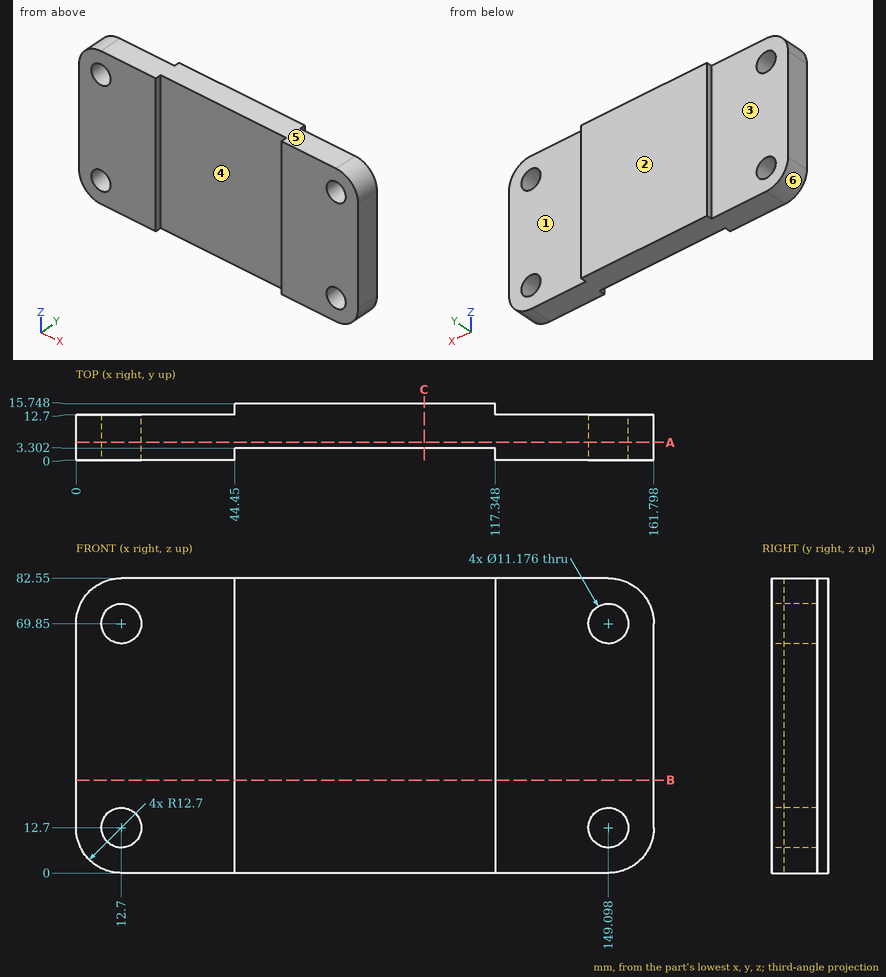
Print and shaded views of the part. All mm, measured from the part's lowest x, y and z. A direction names the side the tool comes from. Give positions to 0.01 mm unless a question says otherwise; leave off trailing zeros. Write each loop counter-clockwise with the first axis right and the second up, starting at its lowest first coordinate (ties: lowest second). Pieces come first, ordered by that corner, then holes. Notation, with made-up numbers: (9.5, -26.5) - (68.5, -26.5) arc R13 cw to (68.5, -4.5) - close; hole circle Ø2 at (70, 63.5). An arc over 180 degrees is marked (long way). Put each result on its own line as item: value.
(1) Saw through at B-B (z = 26). List the corners of the cut face in (x, y), then the cut area to 3 significant figures.
Working result:
outline: (0, 0) - (44.45, 0) - (44.45, 3.3) - (117.35, 3.3) - (117.35, 0) - (161.8, 0) - (161.8, 12.7) - (117.35, 12.7) - (117.35, 15.75) - (44.45, 15.75) - (44.45, 12.7) - (0, 12.7) - close
area: 2,040 mm^2
(2) Tool access for the marked faces 1, 2 and 3: list every direction of +Z, -Z, +X, -X, +Y, -Y with a clear straight run to the whole face (end or side of a thin tool).
Working result:
face 1: +Z, -Z, +X, +Y
face 2: +Z, -Z, +X, -X, +Y
face 3: +Z, -Z, -X, +Y
(3) Pull direction X, two halves, no side cores. Call the marked faces 4, 5 and 6: released by +X, released by -X, zero draft, split by the parting line, or undercut.
Working result:
face 4: undercut
face 5: zero draft
face 6: released by -X
(4) Drop flat-ended pins along their axis: pin 1 Ø10 at (x, z) = (12.7, 69.85) entering from +Y; pin 2 Ø22 at (x, z) = (79, 56) entering from -Y; pin 3 Ø14.5 at (x, z) = (12.7, 12.7) entering from +Y; pin 4 Ø2.5 at (y, z) = (14.5, 23) entering from -X. Give the stop position or say it passes through.
Working result:
pin 1: through
pin 2: y = 3.3
pin 3: y = 12.7
pin 4: x = 44.45
(5) Saw through at C-C (x = 97.5). List the corners of the cut face in (y, z), then the cut area to 3 significant figures.
Working result:
outline: (3.3, 0) - (15.75, 0) - (15.75, 82.55) - (3.3, 82.55) - close
area: 1,030 mm^2
(6) Saw through at A-A (y = 5). List the corners of the cut face in (x, z), then the cut area to 3 significant figures.
Working result:
outline: (0, 12.7) arc R12.7 ccw to (12.7, 0) - (149.1, 0) arc R12.7 ccw to (161.8, 12.7) - (161.8, 69.85) arc R12.7 ccw to (149.1, 82.55) - (12.7, 82.55) arc R12.7 ccw to (0, 69.85) - close; hole circle Ø11.18 at (12.7, 12.7); hole circle Ø11.18 at (12.7, 69.85); hole circle Ø11.18 at (149.1, 12.7); hole circle Ø11.18 at (149.1, 69.85)
area: 12,800 mm^2
(7) Wall check: L1, parallel to X at y = 4, z = 69.85; L2, parallel to X at y = 3, z = 69.85; L3, parallel to X at y = 9, z = 67. Give the ranges that are in metal, low to high.
Working result:
L1: 0 to 7.11, 18.29 to 143.51, 154.69 to 161.8
L2: 0 to 7.11, 18.29 to 44.45, 117.35 to 143.51, 154.69 to 161.8
L3: 0 to 7.89, 17.51 to 144.29, 153.9 to 161.8
